Part model, mm, in its own coordinate system. A direction names the side the tool comes from. Round coordinates to 2 decimals unless told otherwise and drop trailing zeros. Loops run counter-clockwise (first coordinate to the right, second up) from the corner with the lowest first, then second, coordinate; pieces in that order, holes last.
1) Band-saw the part on C-C, the plane y = -20. Write the cut outline in (x, z), then the cut area to 3 significant figures.
2) Band-saw the part on D-D, the plane x = -30. Write the cut outline in (y, z), then the cut area to 3 significant figures.
3) Band-saw the part on B-B, the plane x = -20. Write the cut outline in (y, z), then the cut area to 3 significant figures.
4) Drop flat-ended pins along their axis: P1, Ø1.5, axis at x = 20, y = 2, coming from the +Z side; P2, Ø2.5, axis at x = -28, y = -20.5, coming from the -Z side. Give the stop position or say it passes through.
5) Band-saw the part on A-A, the plane z = 20. Write the cut outline in (x, y), then the cut area to 3 significant figures.
6) 3-axis set-ups, long thin cutter, end or side, ignore diameter. For faces 1 (the flat face through (-40, -1, 8)), 2 (the flat face through (-1, -40, 20)), 3 (the cylindrical face through (-18, 42, 20)), 4 (the cylindrical face through (30.521, -16.034, 3.451)): which of +Z, -Z, +X, -X, +Y, -Y reach the whole face in a straight line?
7) Probe line 1 (X direction, y = 41.9, z = 20); line 2 (Y direction, x = 20, z = 13); line 3 (Z direction, x = 20, y = -43.1). List the from-to ranges inside material, lowest first.
8) Mould opens along X. For faces 5 (the flat face through (40, -1, 8)), 6 (the flat face through (-1, 40, 20)), 7 (the cylindrical face through (-30.521, -23.966, 3.451)), 8 (the flat face through (20, -45, 20)) say: +X half, -X half, draft (parallel to the pull), parting line (faces both ways), or undercut.
from build123d import *

# Parameters (mm, degrees)
SKETCH1_W               = 80
SKETCH1_H               = 100
BOSS_EXTRUDE1_DEPTH     = 10
SKETCH2_R               = 4
CUT_EXTRUDE1_DEPTH      = 7
SKETCH3_W               = 80
SKETCH3_H               = 10
BOSS_EXTRUDE2_DEPTH     = 20
CUT_EXTRUDE2_DEPTH      = 85
CUT_EXTRUDE2_DEPTH_BACK = 5
SKETCH4_R               = 2


with BuildPart() as part:
    # Sketch1 → Boss-Extrude1 (new body)
    with BuildSketch(Plane.XY):
        Rectangle(SKETCH1_W, SKETCH1_H)
    extrude(amount=BOSS_EXTRUDE1_DEPTH)

    # Sketch2 → Cut-Extrude1 (cut)
    with BuildSketch(Plane(origin=(0, 0, 0), x_dir=(-1, 0, 0), z_dir=(0, 0, -1))):
        with Locations((-30, -20)):
            Circle(SKETCH2_R)
        with Locations(Location((30, -20, 0), (0, 0, 180))):
            Circle(SKETCH2_R)
    extrude(amount=-CUT_EXTRUDE1_DEPTH, mode=Mode.SUBTRACT)

    # Sketch3 → Boss-Extrude2 (add)
    with BuildSketch(Plane.XY.offset(10)):
        with Locations((0, -45)):
            Rectangle(SKETCH3_W, SKETCH3_H)
        with Locations((0, 45)):
            Rectangle(SKETCH3_W, SKETCH3_H)
    extrude(amount=BOSS_EXTRUDE2_DEPTH)

    # Sketch4 → Cut-Extrude2 (cut, two sides: drawn at the far end of the back side and taken through both)
    with BuildSketch(Plane(origin=(0, -40, 0), x_dir=(1, 0, 0), z_dir=(0, 1, 0)).offset(-CUT_EXTRUDE2_DEPTH_BACK)):
        with Locations(Location((-20, -20, 0), (0, 0, 270))):
            Circle(SKETCH4_R)
        with Locations(Location((20, -20, 0), (0, 0, 270))):
            Circle(SKETCH4_R)
    extrude(amount=CUT_EXTRUDE2_DEPTH + CUT_EXTRUDE2_DEPTH_BACK, mode=Mode.SUBTRACT)


solid = part.part
Reported:
1. outline: (-40, 0) - (-34, 0) - (-34, 7) - (-26, 7) - (-26, 0) - (26, 0) - (26, 7) - (34, 7) - (34, 0) - (40, 0) - (40, 10) - (-40, 10) - close
1. area: 688 mm2
2. outline: (-50, 0) - (-24, 0) - (-24, 7) - (-16, 7) - (-16, 0) - (50, 0) - (50, 30) - (40, 30) - (40, 10) - (-40, 10) - (-40, 30) - (-50, 30) - close
2. area: 1,340 mm2
3. outline: (-50, 0) - (50, 0) - (50, 30) - (40, 30) - (40, 22) - (45, 22) - (45, 18) - (40, 18) - (40, 10) - (-40, 10) - (-40, 18) - (-45, 18) - (-45, 22) - (-40, 22) - (-40, 30) - (-50, 30) - close
3. area: 1,360 mm2
4. P1: stops at z = 10
4. P2: stops at z = 7
5. outline: (-40, -50) - (40, -50) - (40, -40) - (22, -40) - (22, -45) - (18, -45) - (18, -40) - (-18, -40) - (-18, -45) - (-22, -45) - (-22, -40) - (-40, -40) - close; (-40, 40) - (-22, 40) - (-22, 45) - (-18, 45) - (-18, 40) - (18, 40) - (18, 45) - (22, 45) - (22, 40) - (40, 40) - (40, 50) - (-40, 50) - close
5. area: 1,520 mm2
6. face 1: +Z, -Z, -X, +Y, -Y
6. face 2: +Z, +X, -X
6. face 3: none
6. face 4: -Z
7. line 1: x = -40 to -22, -18 to 18, 22 to 40
7. line 2: y = -50 to -40, 40 to 50
7. line 3: z = 0 to 18, 22 to 30
8. face 5: +X half
8. face 6: draft
8. face 7: undercut
8. face 8: undercut
